Model file for the job. Use its own axes, mm. Face numbers are marked on the shaded views. A direction names the side the tool comes from. Give positions to 0.01 mm unless a question says otherwise; leave off trailing zeros. Use CSV: the item, a comma, the result in double quotes.
from build123d import *

# Parameters (mm, degrees)
SKETCH1_R           = 50.8
SKETCH1_W           = 111.125
SKETCH1_H           = 3.175
BOSS_EXTRUDE1_DEPTH = 38.1
SKETCH2_R           = 6.35
CUT_EXTRUDE1_DEPTH  = 4.445
FILLET1_R           = 3.175


with BuildPart() as part:
    # Sketch1 → Boss-Extrude1 (new, symmetric)
    with BuildSketch(Plane.XY):
        Circle(SKETCH1_R)
        with BuildLine():
            ThreePointArc((-31.929799542, -39.511111111), (-29.93418707, -46.566666667), (-35.921024484, -50.8))
            Line((-35.921024484, -50.8), (7.4e-08, -50.8))
            ThreePointArc((7.4e-08, -50.8), (-16.933333298, -47.894699325), (-31.929799542, -39.511111111))
        make_face()
        with BuildLine():
            Line((7.4e-08, -50.8), (35.921024484, -50.8))
            ThreePointArc((35.921024484, -50.8), (29.93418707, -46.566666667), (31.929799542, -39.511111111))
            ThreePointArc((31.929799542, -39.511111111), (16.933333368, -47.8946993), (7.4e-08, -50.8))
        make_face()
        with Locations((0, -52.3875)):
            Rectangle(SKETCH1_W, SKETCH1_H)
    extrude(amount=BOSS_EXTRUDE1_DEPTH, both=True)

    # Sketch2 → Cut-Extrude1 (cut)
    with BuildSketch(Plane.XY.offset(38.1)):
        Circle(SKETCH2_R)
    extrude(amount=-CUT_EXTRUDE1_DEPTH, mode=Mode.SUBTRACT)

    # Fillet1
    fillet1_edges = [part.edges().sort_by_distance(p)[0] for p in [
        (45.741762242, -50.8, -38.1),
        (45.741762242, -50.8, 38.1),
        (29.93418707, -46.566666667, -38.1),
        (29.93418707, -46.566666667, 38.1),
        (-45.741762242, -50.8, -38.1),
        (-45.741762242, -50.8, 38.1),
        (-29.93418707, -46.566666667, -38.1),
        (-29.93418707, -46.566666667, 38.1),
        (0, 50.8, -38.1),
        (0, 50.8, 38.1),
    ]]
    fillet(fillet1_edges, radius=FILLET1_R - 0.0001)  # a hair under: the kernel refuses the full size


solid = part.part
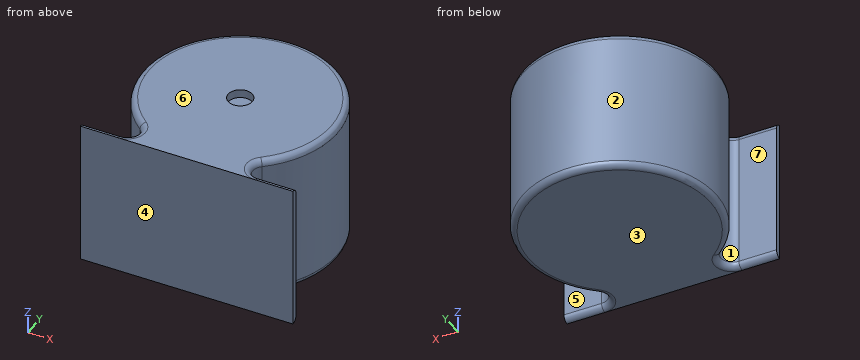
(1) Wall check: probe 1 along Y at (x, z) = (0, 35) (3 decimals); probe 2 along X at (y, z) = (-1.5, 10.5); probe 3 along Y at (x, z) = (41.5, 27) (3 decimals). Give the ranges that are in metal, low to high. Write a range as [from, to].
Checked values:
probe 1,"y = [-53.975, -6.35], [6.35, 50.799]"
probe 2,"x = [-50.78, 50.78]"
probe 3,"y = [-53.975, -50.8], [-29.298, 29.298]"
(2) Pull direction Y, two halves, no side cores. Call the marked faces 1, 2, 3 and 4: released by +Y, released by -Y, zero draft, split by the parting line, or undercut.
Checked values:
face 1,"undercut"
face 2,"undercut"
face 3,"zero draft"
face 4,"released by -Y"
(3) 3-axis set-ups, long thin cutter, end or side, ignore diameter. For the marked faces 5, 6 and 7: which of +Z, -Z, +X, -X, +Y, -Y reach the whole face in a straight line?
Checked values:
face 5,"+Z, -Z, +X"
face 6,"+Z, +X, -X, +Y, -Y"
face 7,"+Z, -Z, -X"
(4) Flat gauge pins, fed straight in: P1, Ø11.5, axis at x = 0, y = 0, coming from the +Z side (3 decimals); P2, Ø15.5, axis at x = 47, z = -1, coming from the +Y side; P3, Ø21.5, axis at x = -46, z = -14, coming from the +Y side. Where does each tip first touch, or does it go through?
Checked values:
P1,"stops at z = 33.655"
P2,"stops at y = 32.25"
P3,"stops at y = 36.58"
